Build history of the part. All positions in model axes, mm. A direction names the side the tool comes from. Round coordinates to 2 decimals unless told otherwise and drop trailing zeros. Loops run counter-clockwise (first coordinate to the right, second up) from the corner with the lowest first, then second, coordinate; pieces in that order, holes last. Notation, with made-up numbers: (26.25, 76.25) -> (68.25, 76.25) arc R23 ccw to (68.25, 110.25) -> close; hole circle Ø3 at (50, 49). An arc over 180 degrees is marked (long way). Put each result on its own line as item: value. Start each with the question number.
Autodesk Inventor part; units mm, degrees
ref_plane "Work Plane1" through (20, 0, 6) normal (0, 0, 1) x (1, 0, 0)
ref_plane "YZ Plane" through (0, 0, 0) normal (1, 0, 0) x (0, 1, 0)
ref_plane "XZ Plane" through (0, 0, 0) normal (0, 1, 0) x (-1, 0, 0)
sketch "Skizze1" plane through (0, 0, 0) normal (0, 0, 1) x (1, 0, 0)
  line L0 (-4, 0) -> (-4, 10)
  line L1 (-4, 10) -> (0, 10)
  line L2 (0, 10) -> (0, 6)
  line L3 (0, 6) -> (40, 6)
  line L4 (40, 6) -> (40, 0)
  line L5 (-4, 0) -> (40, 0)
  line L6 (-4, 0) -> (17, 0)
  line L7 (0, -0.98) -> (0, 3.08)
  circle A0 centre (34.5, 0) radius 1.6
  dimension "d0" = 12
  dimension "d1" = 20
  dimension "d2" = 4
  dimension "d3" = 40
  dimension "d5" = 5.5
  dimension "d6" = 3.2
revolve "Körper" add sketch "Skizze1" angle 360 about axis through (-4, 0, 0) along (1, 0, 0) picked at (34.8992, 0.6089) contours L0 L1 L2 L3 L4 L5 A0 | A0 L5
extrude "Bohrung" cut sketch "Skizze1" along normal through all both and the other way through all contours A0 L5 | L5 A0
chamfer "Fase1" distance 1.6 angle 45 1 edges at (-4, -10, 0) measured on face at (-2.6667, 9.9676, -0.8047)
chamfer "Fase2" distance 3 angle 30 1 edges at (40, -6, 0) measured on face at (13.3333, 5.9805, -0.4828)
ref_plane "Work Plane1" through (20, 0, 6) normal (0, 0, 1) x (1, 0, 0)
equation "\"d0\" = NND"
equation "\"d1\" = KOD"
equation "\"d2\" = KOH"
equation "\"d3\" = NLG"
equation "\"d5\" = DIST"
equation "\"d6\" = BOR"
equation "\"d7\" = NND"
equation "\"d9\" = PHH2"
equation "\"d10\" = FAWI2"
equation "\"d16\" = PHH2"
equation "\"d11\" = PHH1"
equation "\"d12\" = FAWI1"
equation "\"d17\" = PHH1"
equation "\"PHH1\" = 3"
equation "\"PHH2\" = 1.6"
equation "\"KOD\" = 20"
equation "\"KOH\" = 4"
equation "\"NND\" = 12"
equation "\"FAWI1\" = 30deg"
equation "\"FAWI2\" = 45deg"
equation "\"DIST\" = 5.5"
equation "\"BOR\" = 3.2"
equation "\"NLG\" = 40"
properties part number "IS 6863 - B12 x 40" material "Stahl, weich"
Item 1: Cut at C-C on x = 4.5. Write the cut outline in (y, z).
Item 2: Pull direction X, two halves, no side cores. Call faces 1 (the face through (32.9, -0.07, -0.08)), 2 (the face through (-4, 0, 0)), 3 (the face through (-1.18, -2.17, -9.76)), 4 (the face through (0, 7, 0)): +X half, -X half, draft (parallel to the pull), parting line (faces both ways), or undercut.
Item 3: Cut at A-A on y = 0. Write the cut outline in (x, z), then the cut area to 3 significant figures.
Item 4: 3-axis set-ups, long thin cutter, end or side, ignore diameter. For faces 5 (the face through (18.759, 5.723, 1.802)), 6 (the face through (40, 0, 0)): which of +Z, -Z, +X, -X, +Y, -Y reach the whole face in a straight line?
Item 5: Wall check: line 1 (X direction, y = 0, z = 2); line 2 (X direction, y = 4.5, z = -4.5); line 3 (X direction, y = 0.5, z = -4). Give the ranges that are in metal, low to high. Write a range as from..to.
Item 6: Drop flat-ended pins along their axis: pin 1 (1.5 mm diameter, centred on x = 29.5, y = -2, fed in from -Z); pin 2 (1 mm diameter, centred on x = 7.5, y = 2.5, fed in from -Z). Give the stop position or say it passes through.
Item 7: Cut at B-B on z = 0. Write the cut outline in (x, y).
Item 8: Cut at D-D on x = 34.5. Write the cut outline in (y, z).
Ans:
1. outline: circle Ø12 at (0, 0)
2. face 1: undercut
2. face 2: -X half
2. face 3: draft
2. face 4: +X half
3. outline: (-4, -8.4) -> (-2.4, -10) -> (0, -10) -> (0, -6) -> (32.9, -6) -> (32.9, 6) -> (0, 6) -> (0, 10) -> (-2.4, 10) -> (-4, 8.4) -> close; (36.1, -6) -> (37, -6) -> (40, -4.27) -> (40, 4.27) -> (37, 6) -> (36.1, 6) -> close
3. area: 514 mm2
4. face 5: +X
4. face 6: +Z, -Z, +X, +Y, -Y
5. line 1: x = -4..32.9, 36.1..40
5. line 2: x = -4..0
5. line 3: x = -4..32.98, 36.02..40
6. pin 1: stops at z = -5.87
6. pin 2: stops at z = -5.66
7. outline: (-4, -8.4) -> (-2.4, -10) -> (0, -10) -> (0, -6) -> (37, -6) -> (40, -4.27) -> (40, 4.27) -> (37, 6) -> (0, 6) -> (0, 10) -> (-2.4, 10) -> (-4, 8.4) -> close; hole circle Ø3.2 at (34.5, 0)
8. outline: (-1.6, -5.78) -> (-1.6, 5.78) arc R6 ccw to start; (1.6, -5.78) arc R6 ccw to (1.6, 5.78) -> close
